```python
from build123d import *

# Parameters (mm, degrees)
SALIENTE_EXTRUIR1_DEPTH           = 40
CROQUIS2_W                        = 40
CROQUIS2_H                        = 80
SALIENTE_EXTRUIR2_DEPTH           = 50
CORTAR_EXTRUIR1_DEPTH             = 41
CROQUIS4_W                        = 25.000000038
CROQUIS4_H                        = 50
CORTAR_EXTRUIR2_DEPTH             = 41
DI_METRO_DE_TALADRO_5_0_5_1_D     = 5
DI_METRO_DE_TALADRO_5_0_5_1_DEPTH = 25.000025
DI_METRO_DE_TALADRO_5_0_5_2_D     = 5
DI_METRO_DE_TALADRO_5_0_5_2_DEPTH = 40.00005
DI_METRO_DE_TALADRO_5_0_5_3_D     = 5
DI_METRO_DE_TALADRO_5_0_5_3_DEPTH = 90.000025


with BuildPart() as part:
    # Croquis1 → Saliente-Extruir1 (new body)
    with BuildSketch(Plane(origin=(-40, 0, 0), x_dir=(0, -1, 0), z_dir=(-1, 0, 0))):
        Polygon((-37.940430416, 40), (-37.940430416, -25), (52.059569584, -25), (42.059569584, 0), (42.059569584, 40), align=None)
    extrude(amount=-SALIENTE_EXTRUIR1_DEPTH)

    # Croquis2 → Saliente-Extruir2 (add)
    with BuildSketch(Plane(origin=(0, 0, -25), x_dir=(-1, 0, 0), z_dir=(0, 0, -1))):
        with Locations((20, -2.059569584)):
            Rectangle(CROQUIS2_W, CROQUIS2_H)
    extrude(amount=SALIENTE_EXTRUIR2_DEPTH)

    # Croquis3 → Cortar-Extruir1 (cut, through all)
    with BuildSketch(Plane.ZY.offset(40)):
        with BuildLine():
            ThreePointArc((-32.5, -22.059569584), (-30, -24.559569584), (-27.5, -22.059569584))
            ThreePointArc((-27.5, -22.059569584), (-13.587572106, 11.528002522), (20, 25.440430416))
            ThreePointArc((20, 25.440430416), (22.5, 27.940430416), (20, 30.440430416))
            ThreePointArc((20, 30.440430416), (-17.123106012, 15.063536428), (-32.5, -22.059569584))
        make_face()
    extrude(amount=-CORTAR_EXTRUIR1_DEPTH, mode=Mode.SUBTRACT)

    # Croquis4 → Cortar-Extruir2 (cut, through all)
    with BuildSketch(Plane(origin=(0, 0, 0), x_dir=(0, 0, -1), z_dir=(1, 0, 0))):
        with Locations((52.499999981, -2.059569584)):
            Rectangle(CROQUIS4_W, CROQUIS4_H)
    extrude(amount=-CORTAR_EXTRUIR2_DEPTH, mode=Mode.SUBTRACT)

    # Diámetro de taladro Ø5.0 (5)1
    with Locations(Plane(origin=(0, -27.059569584, 0), x_dir=(1, 0, 0), z_dir=(0, 1, 0))):
        with Locations((-20, 55)):
            Hole(DI_METRO_DE_TALADRO_5_0_5_1_D / 2, depth=DI_METRO_DE_TALADRO_5_0_5_1_DEPTH)

    # Diámetro de taladro Ø5.0 (5)2
    with Locations(Plane(origin=(0, 0, 0), x_dir=(0, 0, -1), z_dir=(1, 0, 0))):
        with Locations((-20, -22.059569584)):
            Hole(DI_METRO_DE_TALADRO_5_0_5_2_D / 2, depth=DI_METRO_DE_TALADRO_5_0_5_2_DEPTH)

    # Diámetro de taladro Ø5.0 (5)3
    with Locations(Plane(origin=(0, 37.940430416, 0), x_dir=(1, 0, 0), z_dir=(0, 1, 0))):
        with Locations((-20, 55)):
            Hole(DI_METRO_DE_TALADRO_5_0_5_3_D / 2, depth=DI_METRO_DE_TALADRO_5_0_5_3_DEPTH)


solid = part.part
```
Geometry check sheet. Reference: the model listing, model coordinates, mm. A direction names the side the tool comes from. Coordinates: 2 decimals unless noted, no trailing zeros. Loops run counter-clockwise (first coordinate to the right, second up) from the corner with the lowest first, then second, coordinate; pieces in that order, holes last.
Item 1: Thickness scan on line 1 (Y direction, x = -31, z = 20); line 2 (X direction, y = 32.75, z = -55); line 3 (Z direction, x = -22.5, y = -26). Record the ranges inside material, lowest first.
Item 2: Sectioned sample at D-D, the plane x = -6. Record the boundary of the cut face in (y, z), then the cut area to 3 significant figures.
Item 3: Access from +Z, -Z, +X, -X, +Y, -Y to the whole of each face (thin tool, end or side, straight path). Record for faces 1 (the face through (-20, -42.06, 20)), 2 (the face through (-20, -42.06, -50)), 3 (the face through (-20, -3, 40)), 4 (the face through (-20, -27.06, -52)).
Item 4: Sectioned sample at A-A, the plane x = -20. Record the boundary of the cut face in (y, z).
Item 5: Go/stop test with flat-tipped pins: pin 1 Ø5 at (x, y) = (-15.5, -45) entering from -Z; pin 2 Ø12 at (x, z) = (-18, -55.5) entering from -Y. Record where each tip stops, or that it passes through.
Item 6: Sectioned sample at B-B, the plane z = -55. Record the boundary of the cut face in (x, y).
Item 7: Sectioned sample at C-C, the plane y = -8.5. Record the boundary of the cut face in (x, z).
Item 8: Release check for a two-part mould opening along Y. For faces 5 (the face through (-20, -47, -25)), 6 (the face through (-20.28, -21.95, 17.502)), 7 (the face through (-20.28, -47.13, -12.68)) record: released by +Y, released by -Y, zero draft, split by the parting line, or undercut.
Check result:
1. line 1: y = -42.06 to -24.56, -19.56 to 25.44, 30.44 to 37.94
1. line 2: x = -40 to -22.5, -17.5 to 0
1. line 3: z = -75 to -65, -40 to 40
2. outline: (-52.06, -25) - (-42.06, -25) - (-42.06, -75) - (37.94, -75) - (37.94, 40) - (-42.06, 40) - (-42.06, 0) - close; hole (-27.06, -65) - (22.94, -65) - (22.94, -40) - (-27.06, -40) - close; hole circle Ø5 at (-22.06, 20); hole (-22.06, -32.5) arc R52.5 ccw to (30.44, 20) arc R2.5 ccw to (25.44, 20) arc R47.5 cw to (-22.06, -27.5) arc R2.5 ccw to start
2. area: 7,640 mm2
3. face 1: +Z, +X, -X, -Y
3. face 2: -Z, +X, -X, -Y
3. face 3: +Z, +X, -X, +Y, -Y
3. face 4: +X, -X
4. outline: (-52.06, -25) - (-42.06, -25) - (-42.06, -52.5) - (-27.06, -52.5) - (-27.06, -40) - (22.94, -40) - (22.94, -52.5) - (37.94, -52.5) - (37.94, 40) - (-42.06, 40) - (-42.06, 0) - close; (-42.06, -75) - (37.94, -75) - (37.94, -57.5) - (22.94, -57.5) - (22.94, -65) - (-27.06, -65) - (-27.06, -57.5) - (-42.06, -57.5) - close; hole circle Ø5 at (-22.06, 20); hole (-22.06, -32.5) arc R52.5 ccw to (30.44, 20) arc R2.5 ccw to (25.44, 20) arc R47.5 cw to (-22.06, -27.5) arc R2.5 ccw to start
5. pin 1: stops at z = -25
5. pin 2: stops at y = -42.06
6. outline: (-40, -42.06) - (-22.5, -42.06) - (-22.5, -27.06) - (-40, -27.06) - close; (-40, 22.94) - (-22.5, 22.94) - (-22.5, 37.94) - (-40, 37.94) - close; (-17.5, -42.06) - (0, -42.06) - (0, -27.06) - (-17.5, -27.06) - close; (-17.5, 22.94) - (0, 22.94) - (0, 37.94) - (-17.5, 37.94) - close
7. outline: (-40, -75) - (0, -75) - (0, -65) - (-40, -65) - close; (-40, -40) - (0, -40) - (0, -30.72) - (-40, -30.72) - close; (-40, -25.52) - (0, -25.52) - (0, 40) - (-40, 40) - close
8. face 5: zero draft
8. face 6: undercut
8. face 7: released by -Y
